Work out the finished part from the listing and answer in its coordinate system (mm). A direction names the side the tool comes from. Round coordinates to 2 decimals unless told otherwise and drop trailing zeros. Loops run counter-clockwise (first coordinate to the right, second up) from the corner with the lowest first, then second, coordinate; pieces in that order, holes last. Notation, with made-up numbers: (16.5, 22) - (32.5, 22) arc R4 cw to (32.5, 26) - close; hole circle Ø9 at (3.25, 67). An arc over 180 degrees is marked (long way). Answer as CSV lines item,"result". Start each with the question number.
```python
from build123d import *

# Parameters (mm, degrees)
SKETCH1_R               = 7.5
BOSS_EXTRUDE1_DEPTH     = 10
SKETCH2_R               = 30
BOSS_EXTRUDE2_DEPTH     = 65
CUT_EXTRUDE1_DEPTH      = 121.933866224
CUT_EXTRUDE1_DEPTH_BACK = 121.933866224
SKETCH3_W               = 15
SKETCH3_H               = 65
SKETCH5_W               = 12.5
SKETCH5_H               = 30
CUT_EXTRUDE2_DEPTH      = 121.933866224


with BuildPart() as part:
    # Sketch1 → Boss-Extrude1 (new body)
    with BuildSketch(Plane(origin=(0, 0, 0), x_dir=(1, 0, 0), z_dir=(0, 1, 0))):
        with BuildLine():
            Line((6, 29.393876913), (78, 14.696938457))
            ThreePointArc((78, 14.696938457), (90, 0), (78, -14.696938457))
            Line((78, -14.696938457), (6, -29.393876913))
            ThreePointArc((6, -29.393876913), (0, -30), (-6, -29.393876913))
            Line((-6, -29.393876913), (-78, -14.696938457))
            ThreePointArc((-78, -14.696938457), (-90, 0), (-78, 14.696938457))
            Line((-78, 14.696938457), (-6, 29.393876913))
            ThreePointArc((-6, 29.393876913), (0, 30), (6, 29.393876913))
        make_face()
        with Locations(Location((-75, 0, 0), (0, 0, 270))):
            Circle(SKETCH1_R, mode=Mode.SUBTRACT)
        with Locations(Location((75, 0, 0), (0, 0, 270))):
            Circle(SKETCH1_R, mode=Mode.SUBTRACT)
    extrude(amount=BOSS_EXTRUDE1_DEPTH)

    # Sketch2 → Boss-Extrude2 (add)
    with BuildSketch(Plane(origin=(0, 10, 0), x_dir=(1, 0, 0), z_dir=(0, 1, 0))):
        with Locations(Location((0, 0, 0), (0, 0, 78.463040967))):
            Circle(SKETCH2_R)
    extrude(amount=BOSS_EXTRUDE2_DEPTH)

    # Sketch3 → Cut-Extrude1 (cut, two sides: drawn at the far end of the back side and taken through both)
    with BuildSketch(Plane(origin=(0, 0, 0), x_dir=(0, 0, -1), z_dir=(1, 0, 0)).offset(-CUT_EXTRUDE1_DEPTH_BACK)):
        with Locations((0, 42.5)):
            Rectangle(SKETCH3_W, SKETCH3_H)
    extrude(amount=CUT_EXTRUDE1_DEPTH + CUT_EXTRUDE1_DEPTH_BACK, mode=Mode.SUBTRACT)

    # Sketch5 → Cut-Extrude2 (cut, symmetric)
    with BuildSketch(Plane(origin=(0, 0, 0), x_dir=(0, 0, -1), z_dir=(1, 0, 0))):
        with Locations((-23.75, 60)):
            Rectangle(SKETCH5_W, SKETCH5_H)
    cut_extrude2 = extrude(amount=CUT_EXTRUDE2_DEPTH, both=True, mode=Mode.SUBTRACT)

    # Mirror1: Cut-Extrude2 across plane
    add(cut_extrude2.mirror(Plane.XY), mode=Mode.SUBTRACT)


solid = part.part
```
Item 1: Section D-D, the plane y = 39.5 is taken. Give the vertices of the cut face in (x, z), and give its area (3 significant figures).
Item 2: Which of the six approach directions +Z, -Z, +X, -X, +Y, -Y give full straight-line access (tool end or side, diameter ignored) to faces 4 (the face through (1, 10, 0)), 5 (the face through (0, 45, -22)), 6 (the face through (0, 60, 17.5)), 7 (the face through (-81.654, 4.93, 3.461)), 8 (the face through (0, 42, 7.5))?
Item 3: Section C-C, the plane x = -75 is taken. Give the vertices of the cut face in (y, z), and give its area (3 significant figures).
Item 4: Section A-A, the plane z = 0 is taken. Give the vertices of the cut face in (x, y), and give its area (3 significant figures).
Item 5: Find the intervals of material crossed by L1, parallel to X at y = 5, z = 0; L2, parallel to Z at x = 0, y = 14; L3, parallel to Y at x = -26, z = -1, in increasing order.
Item 6: Determine the mould class of faces 1 (the face through (90, 5, 0)), 2 (the face through (0, 42, -7.5)), 3 (the face through (0, 45, 22)) for opening direction Z: pulls with the +Z half, pulls with the -Z half, needs draft (parallel to the pull), parting line crosses it, or undercut.
Item 7: Section B-B, the plane y = 5 is taken. Give the vertices of the cut face in (x, z), and give its area (3 significant figures).
Item 8: Flat-ended cylindrical pins translate along their axes: pin 1 Ø24 at (x, y) = (0, 65.5) entering from -Z; pin 2 Ø10 at (x, z) = (4.5, 26) entering from +Y; pin 3 Ø5 at (y, z) = (15, -8.5) entering from +X. Find the tip coordinate at first contact, or state that the pin passes through.
Answer:
1,outline,"(-29.05, -7.5) arc R30 ccw to (29.05, -7.5) - close; (-29.05, 7.5) - (29.05, 7.5) arc R30 ccw to start"
1,area,"1,940 mm²"
2,face 4,"+Y"
2,face 5,"-Z, +X, -X, +Y"
2,face 6,"+Z, +X, -X, +Y"
2,face 7,"+Y, -Y"
2,face 8,"+X, -X, +Y"
3,outline,"(0, -15.31) - (10, -15.31) - (10, -7.5) - (0, -7.5) - close; (0, 7.5) - (10, 7.5) - (10, 15.31) - (0, 15.31) - close"
3,area,"156 mm²"
4,outline,"(-90, 0) - (-82.5, 0) - (-82.5, 10) - (-90, 10) - close; (-67.5, 0) - (67.5, 0) - (67.5, 10) - (-67.5, 10) - close; (82.5, 0) - (90, 0) - (90, 10) - (82.5, 10) - close"
4,area,"1,500 mm²"
5,L1,"x = -90 to -82.5, -67.5 to 67.5, 82.5 to 90"
5,L2,"z = -30 to -7.5, 7.5 to 30"
5,L3,"y = 0 to 10"
6,face 1,"parting line crosses it"
6,face 2,"undercut"
6,face 3,"needs draft"
7,outline,"(-78, -14.7) - (-6, -29.39) arc R30 ccw to (6, -29.39) - (78, -14.7) arc R15 ccw to (78, 14.7) - (6, 29.39) arc R30 ccw to (-6, 29.39) - (-78, 14.7) arc R15 ccw to start; hole circle Ø15 at (-75, 0); hole circle Ø15 at (75, 0)"
7,area,"7,240 mm²"
8,pin 1,"stops at z = -17.5"
8,pin 2,"stops at y = 45"
8,pin 3,"stops at x = 29.05"
